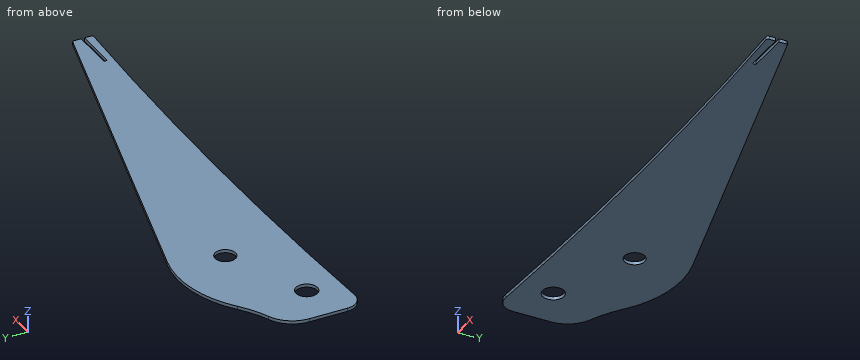
```python
from build123d import *

# Parameters (mm, degrees)
BOSS_EXTRUDE1_DEPTH = 3
SKETCH2_R           = 9.5
CUT_EXTRUDE2_DEPTH  = 456.583037544
SKETCH6_W           = 40
SKETCH6_H           = 3
CUT_EXTRUDE4_DEPTH  = 456.583037544
SKETCH7_R           = 10
CUT_EXTRUDE5_DEPTH  = 10


with BuildPart() as part:
    # Sketch1 → Boss-Extrude1 (new body)
    with BuildSketch(Plane.XY):
        with BuildLine():
            Line((108.154123351, 67.552328068), (448.523707095, -24.796940542))
            ThreePointArc((448.523707095, -24.796940542), (449.588617983, -25.51212784), (450, -26.727155784))
            Line((450, -26.727155784), (450, -42.109493017))
            ThreePointArc((450, -42.109493017), (449.373989907, -43.562817391), (447.887848264, -44.106346038))
            ThreePointArc((447.887848264, -44.106346038), (219.361402367, -37.652818923), (-9.169620431, -43.942183392))
            ThreePointArc((-9.169620431, -43.942183392), (-20.308838598, -39.861416221), (-25, -28.96518537))
            Line((-25, -28.96518537), (-25, 6.26137734))
            ThreePointArc((-25, 6.26137734), (-19.871474725, 23.036649171), (-6.239350333, 34.076427296))
            ThreePointArc((-6.239350333, 34.076427296), (7.186208551, 40.672066088), (19.515669553, 49.14156866))
            ThreePointArc((19.515669553, 49.14156866), (61.632192327, 68.951849742), (108.154123351, 67.552328068))
        make_face()
    extrude(amount=BOSS_EXTRUDE1_DEPTH)

    # Sketch2 → Cut-Extrude2 (cut, through all)
    with BuildSketch(Plane.XY.offset(3)):
        with Locations((94.5, 21)):
            Circle(SKETCH2_R)
    extrude(amount=-CUT_EXTRUDE2_DEPTH, mode=Mode.SUBTRACT)

    # Sketch6 → Cut-Extrude4 (cut, through all)
    with BuildSketch(Plane.XY.offset(3)):
        with Locations((430, -34.843289866)):
            Rectangle(SKETCH6_W, SKETCH6_H)
    extrude(amount=-CUT_EXTRUDE4_DEPTH, mode=Mode.SUBTRACT)

    # Sketch7 → Cut-Extrude5 (cut)
    with BuildSketch(Plane.XY.offset(3)):
        with Locations((15.211776531, -12.474975597)):
            Circle(SKETCH7_R)
    extrude(amount=-CUT_EXTRUDE5_DEPTH, mode=Mode.SUBTRACT)


solid = part.part
```
Geometry: final body of the model. Coordinates: model frame, mm. Round coordinates to 2 decimals unless told otherwise and drop trailing zeros. Loops run counter-clockwise (first coordinate to the right, second up) from the corner with the lowest first, then second, coordinate; pieces in that order, holes last. Notation, with made-up numbers: (33.5, 61) -> (49.5, 61) arc R30 ccw to (49.5, 90) -> close; hole circle Ø7 at (-2.5, 61.25). An arc over 180 degrees is marked (long way). Use one line per item in the form item = value. Start each with the question number.
1) Section D-D on x = 336.5. Output: boundary loops of the cut face in (y, z), then the cut area to 3 significant figures.
2) Section B-B on x = 94.5. Output: boundary loops of the cut face in (y, z).
3) Section A-A on y = 21. Output: boundary loops of the cut face in (x, z), then the cut area to 3 significant figures.
4) Section C-C on z = 1.45. Output: boundary loops of the cut face in (x, y).
5) First-contact query: P1, Ø1, axis at x = 301.5, z = 2.5, coming from the +Y side. Flat tip, straight axial feed; report the tip coordinate or a pass-through.
6) Line query: L1, parallel to Y at x = 94.5, z = 2; L2, parallel to X at y = -31.5, z = 2.6; L3, parallel to Y at x = 28, z = 1. Output: solid intervals per line, ascending.
Response:
q1.outline = (-39.37, 0) -> (5.6, 0) -> (5.6, 3) -> (-39.37, 3) -> close
q1.area = 135 mm^2
q2.outline = (-39.51, 0) -> (11.5, 0) -> (11.5, 3) -> (-39.51, 3) -> close; (30.5, 0) -> (70.25, 0) -> (70.25, 3) -> (30.5, 3) -> close
q3.outline = (-21.13, 0) -> (85, 0) -> (85, 3) -> (-21.13, 3) -> close; (104, 0) -> (279.73, 0) -> (279.73, 3) -> (104, 3) -> close
q3.area = 846 mm^2
q4.outline = (-25, -28.97) arc R15 ccw to (-9.17, -43.94) arc R4101.58 cw to (447.89, -44.11) arc R2 ccw to (450, -42.11) -> (450, -36.34) -> (410, -36.34) -> (410, -33.34) -> (450, -33.34) -> (450, -26.73) arc R2 ccw to (448.52, -24.8) -> (108.15, 67.55) arc R100 ccw to (19.52, 49.14) arc R103.07 cw to (-6.24, 34.08) arc R30 ccw to (-25, 6.26) -> close; hole circle Ø20 at (15.21, -12.47); hole circle Ø19 at (94.5, 21)
q5.P1 = 15.23
q6.L1 = -39.51 to 11.5, 30.5 to 70.25
q6.L2 = -24.78 to 450
q6.L3 = -42.05 to 55.23
